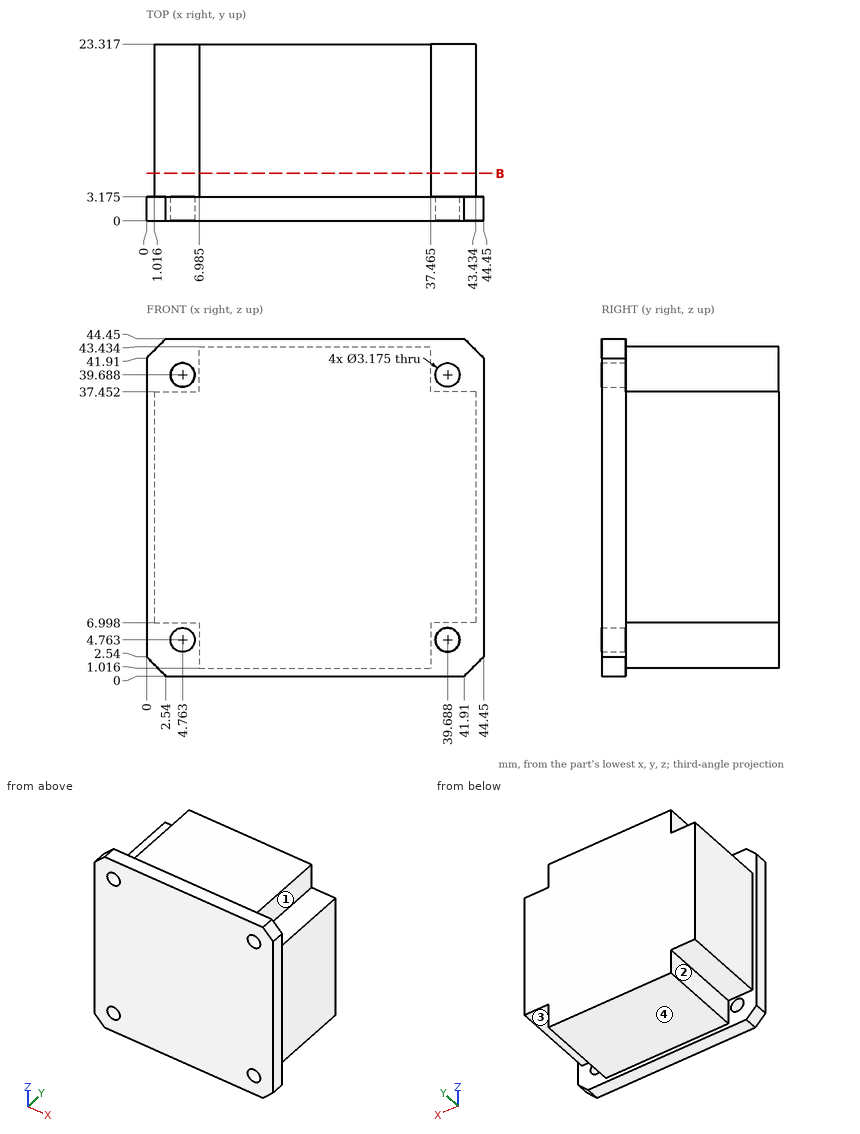
Input: dimensioned drawing with shaded views. Units: mm. Origin: part minimum x, y, z. A direction names the side the tool comes from. Round coordinates to 2 decimals unless told otherwise and drop trailing zeros. Order: outer loops, then holes, each group sorted by start corner. A loop starts at its lowest first (then second) coordinate and runs counter-clockwise, first axis right, second up. Notation, with made-up numbers: (-30.5, 82) -> (-10.5, 82) arc R19 cw to (-10.5, 92) -> close; hole circle Ø1 at (-8.5, 3). An arc over 180 degrees is marked (long way). One line per item, written item: value. Start each with the question number.
Q1. Section query B-B (y = 6.25). Return the cut outline in (x, z) (1 decimal).
Q2. Access query for the marked faces 1, 2, 3 and 4. Directions: +Z, -Z, +X, -X, +Y, -Y. A direction counts if a zero-diameter tool reaches every point of the face in a straight line with its end or side. Return the directions, or none.
Q3. Pin query (flat end, axial travel): pin 1 (5 mm diameter, centred on x = 28, y = 8, fed in from +Z); pin 2 (6.5 mm diameter, centred on y = 15.5, z = 39.5, fed in from +X); pin 3 (5 mm diameter, centred on x = 42, y = 11.5, fed in from +Z). Return the tip coordinate at first contact, or that it passes through.
Q4. Material intervals for probe 1 along Z at (x, y) = (30, 12.5) (1 decimal); probe 2 along X at (y, z) = (16.75, 5) (1 decimal), sorted ascending.
Findings below:
1. outline: (1, 7) -> (7, 7) -> (7, 1) -> (37.5, 1) -> (37.5, 7) -> (43.4, 7) -> (43.4, 37.5) -> (37.5, 37.5) -> (37.5, 43.4) -> (7, 43.4) -> (7, 37.5) -> (1, 37.5) -> close
2. face 1: +Z, +X, +Y
2. face 2: -Z, -X, +Y
2. face 3: -Z, +X, +Y
2. face 4: -Z, +X, -X, +Y
3. pin 1: z = 43.43
3. pin 2: x = 43.43
3. pin 3: z = 37.45
4. probe 1: 1 to 43.4
4. probe 2: 7 to 37.5
